CAD build for the part. Positions are in the model's coordinates, mm. Face numbers are marked on the shaded views. Round coordinates to 2 decimals unless told otherwise and drop trailing zeros. Write each loop counter-clockwise with the first axis right and the second up, starting at its lowest first coordinate (ties: lowest second). Pieces come first, ordered by that corner, then holes. Notation, with made-up numbers: (15, 56.5) - (58, 56.5) arc R22 ccw to (58, 79.5) - close; hole circle Ø6 at (5.25, 2.25). An arc over 180 degrees is marked (long way). Put each result on its own line as item: value. Start each with the question number.
Item 1: Cut at B-B (z = 10.75). Count the separate pieces of the cut face and the enclosed holes in it, and give its area (3 significant figures).
Item 2: Cut at A-A (x = 0). Give the cut face in (y, z), and give its area (3 significant figures).
Item 3: Pin check, flat tips, straight feed: pin 1 Ø8 at (x, y) = (120, 0) entering from +Z; pin 2 Ø6.5 at (x, y) = (-36, -11.5) entering from +Z. Stop position of each tip, or through.
Item 4: Mould opens along Y. For the marked faces 1, 2 and 3 say: released by +Y, released by -Y, zero draft, split by the parting line, or undercut.
Item 5: Drill centre lines: line 1 (Y direction, x = 36, z = 8.25); line 2 (Y direction, x = 0, z = 10.75); line 3 (X direction, y = -2, z = 5). Where is each one in solid material? Low to high. Write a range as from..to.
Item 6: Cut at C-C (x = -120). Give the cut face in (y, z).
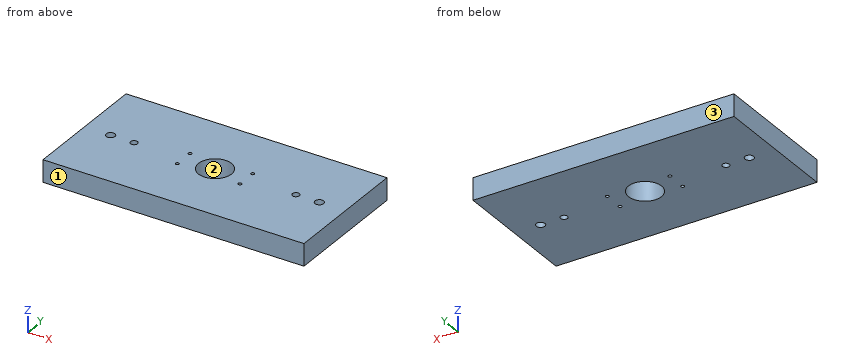
Autodesk Inventor part; units mm, degrees
ref_plane "YZ Plane" through (0, 0, 0) normal (1, 0, 0) x (0, 1, 0)
ref_plane "XZ Plane" through (0, 0, 0) normal (0, 1, 0) x (-1, 0, 0)
ref_plane "XY Plane" through (0, 0, 0) normal (0, 0, 1) x (1, 0, 0)
sketch "Sketch1" plane through (0, 0, 0) normal (0, 0, 1) x (1, 0, 0)
  line L0 (-150, -75) -> (150, -75)
  line L1 (150, -75) -> (150, 75)
  line L2 (150, 75) -> (-150, 75)
  line L3 (-150, 75) -> (-150, -75)
  line L4 (-150, -75) -> (150, 75) construction
  line L5 (150, -75) -> (-150, 75) construction
  point P0 (0, 0)
  dimension "d0" = 300
  dimension "d1" = 150
extrude "Extrusion1" add sketch "Sketch1" along normal blind 25.4
sketch "Sketch2" plane through (0, 0, 25.4) normal (0, 0, 1) x (1, 0, 0)
  line L0 (-120, 0) -> (120, 0)
  line L1 (-150, 75) -> (-150, -75)
  point P0 (0, 0)
  point P1 (0, 0)
  dimension "d4" = 30
hole "Hole1" at (-120, 0, 25.4) at (120, 0, 25.4) direction (0, 0, -1) diameter 10 end through all
sketch "Sketch3" plane through (0, 0, 25.4) normal (0, 0, 1) x (1, 0, 0)
  line L0 (-93, 0) -> (93, 0)
  point P0 (0, 0)
  point P1 (0, 0)
  dimension "d26" = 186
hole "Hole2" at (-93, 0, 25.4) at (93, 0, 25.4) direction (0, 0, -1) diameter 8 end through all
sketch "Sketch4" plane through (0, 0, 25.4) normal (0, 0, 1) x (1, 0, 0)
  point P0 (0, 0)
  point P1 (0, 0)
hole "Hole3" at (0, 0, 25.4) direction (0, 0, -1) diameter 38.1 end through all
sketch "Sketch5" plane through (0, 0, 25.4) normal (0, 0, 1) x (1, 0, 0)
  circle A0 centre (-36, 11.5) radius 2
  line L0 (-150, 75) -> (-150, -75) construction
  line L1 (-150, 0) -> (150, 0) construction
  line L2 (150, -75) -> (150, 75) construction
  circle A1 centre (-36, -11.5) radius 2
  line L3 (150, 75) -> (-150, 75) construction
  line L4 (0, 75) -> (0, -75) construction
  line L5 (-150, -75) -> (150, -75) construction
  circle A2 centre (36, 11.5) radius 2
  circle A3 centre (36, -11.5) radius 2
  point P0 (0, 0)
  dimension "d27" = 4
  dimension "d28" = 36
  dimension "d29" = 11.5
extrude "Extrusion2" cut sketch "Sketch5" against normal up to next
properties part number "base de madera pequeña"
Output values:
1. separate pieces: 1
1. enclosed holes: 9
1. area: 43,600 mm2
2. outline: (-75, 0) - (-19.05, 0) - (-19.05, 25.4) - (-75, 25.4) - close; (19.05, 0) - (75, 0) - (75, 25.4) - (19.05, 25.4) - close
2. area: 2,840 mm2
3. pin 1: through
3. pin 2: z = 25.4
4. face 1: released by -Y
4. face 2: undercut
4. face 3: released by +Y
5. line 1: -75..-13.5, -9.5..9.5, 13.5..75
5. line 2: -75..-19.05, 19.05..75
5. line 3: -150..-124.58, -115.42..-96.46, -89.54..-18.94, 18.94..89.54, 96.46..115.42, 124.58..150
6. outline: (-75, 0) - (-5, 0) - (-5, 25.4) - (-75, 25.4) - close; (5, 0) - (75, 0) - (75, 25.4) - (5, 25.4) - close
